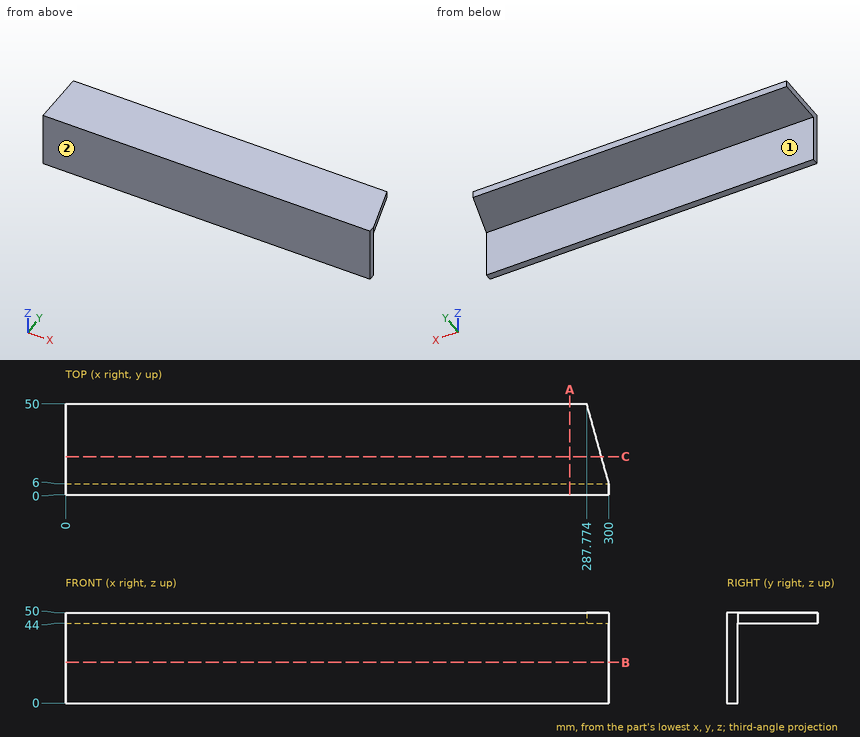
Source: three-view drawing plus pictorial views. Frame: mm from the lowest corner of the part. A direction names the side the tool comes from. Round coordinates to 2 decimals unless told otherwise and drop trailing zeros. Loops run counter-clockwise (first coordinate to the right, second up) from the corner with the lowest first, then second, coordinate; pieces in that order, holes last.
Q1. Section C-C on y = 21. Return loops of the section in (x, z).
Q2. Section B-B on z = 22.5. Return loops of the section in (x, y), plus the area to 3 significant figures.
Q3. Material intervals for L1, parallel to Z at x = 212.5, y = 24.5; L2, parallel to Y at x = 163.5, z = 35; L3, parallel to X at y = 46.5, z = 46 (1 decimal), sorted ascending.
Q4. Pin query (flat end, axial travel): P1, Ø1.5, axis at x = 69.5, y = 17.5, coming from the -Z side; P2, Ø1.5, axis at x = 236.5, z = 6, coming from the +Y side. Return the tip coordinate at first contact, or that it passes through.
Q5. Section A-A on x = 278.5. Return loops of the section in (y, z).
Q6. Access query for the marked faces 1 and 2. Directions: +Z, -Z, +X, -X, +Y, -Y. A direction counts if a zero-diameter tool reaches every point of the face in a straight line with its end or side. Return the directions, or none.
Evaluation:
1. outline: (0, 44) - (295.83, 44) - (295.83, 50) - (0, 50) - close
2. outline: (0, 0) - (300, 0) - (300, 6) - (0, 6) - close
2. area: 1,800 mm2
3. L1: z = 44 to 50
3. L2: y = 0 to 6
3. L3: x = 0 to 288.7
4. P1: stops at z = 44
4. P2: stops at y = 6
5. outline: (0, 0) - (6, 0) - (6, 44) - (50, 44) - (50, 50) - (0, 50) - close
6. face 1: -Z, +X, -X, +Y
6. face 2: +Z, -Z, +X, -X, -Y
